from build123d import *

# Parameters (mm, degrees)
BOSS_EXTRUDE2_DEPTH = 15
SKETCH3_R           = 27
BOSS_EXTRUDE3_DEPTH = 46
SKETCH4_R           = 36
BOSS_EXTRUDE4_DEPTH = 38
MIRROR3_START       = 175
MIRROR3_OUTLINE_R   = 36
MIRROR3_DEPTH       = 53
MIRROR3_START_2     = 114
MIRROR3_2_DEPTH     = 15
MIRROR3_3_OUTLINE_R = 36
MIRROR3_3_DEPTH     = 15
MIRROR3_START_3     = 129
MIRROR3_4_OUTLINE_R = 27
MIRROR3_4_DEPTH     = 46


# Read off the part's stored shape, not the designer's step: Mirror3
with BuildPart() as part:
    # Sketch2 → Boss-Extrude2 (new body)
    with BuildSketch(Plane.XY):
        with BuildLine():
            Line((64.569893475, 47.23059238), (34.517510455, -54.224552409))
            ThreePointArc((34.517510455, -54.224552409), (0, -80), (-34.517510455, -54.224552409))
            Line((-34.517510455, -54.224552409), (-64.569893475, 47.23059238))
            ThreePointArc((-64.569893475, 47.23059238), (0, 80), (64.569893475, 47.23059238))
        make_face()
    boss_extrude2 = extrude(amount=BOSS_EXTRUDE2_DEPTH)

    # Sketch3 → Boss-Extrude3 (add)
    with BuildSketch(Plane.XY.offset(15)):
        with Locations((0, -44)):
            Circle(SKETCH3_R)
    extrude(amount=BOSS_EXTRUDE3_DEPTH)

    # Sketch4 → Boss-Extrude4 (add)
    with BuildSketch(Plane(origin=(0, 0, 0), x_dir=(-1, 0, 0), z_dir=(0, 0, -1))):
        Circle(SKETCH4_R)
    boss_extrude4 = extrude(amount=BOSS_EXTRUDE4_DEPTH)

    # Mirror2: Boss-Extrude2, Boss-Extrude4 across plane
    add(boss_extrude2.mirror(Plane.XY.offset(38)))
    add(boss_extrude4.mirror(Plane.XY.offset(38)))

    # Mirror3 2 outline → Mirror3 2 (add)
    with BuildSketch(Plane.XY.offset(MIRROR3_START_2)):
        with BuildLine():
            Line((-64.569893475, 47.23059238), (-34.517510455, -54.224552409))
            ThreePointArc((-34.517510455, -54.224552409), (0, -80), (34.517510455, -54.224552409))
            Line((34.517510455, -54.224552409), (64.569893475, 47.23059238))
            ThreePointArc((64.569893475, 47.23059238), (0, 80), (-64.569893475, 47.23059238))
        make_face()
    extrude(amount=MIRROR3_2_DEPTH)



with BuildPart() as body_2:
    # Mirror3 outline → Mirror3 (new body)
    with BuildSketch(Plane.XY.offset(MIRROR3_START)):
        Circle(MIRROR3_OUTLINE_R)
    extrude(amount=MIRROR3_DEPTH)

    # Mirror3 3 outline → Mirror3 3 (add)
    with BuildSketch(Plane.XY.offset(MIRROR3_START)):
        with BuildLine():
            Line((-64.569893475, 47.23059238), (-34.517510455, -54.224552409))
            ThreePointArc((-34.517510455, -54.224552409), (0, -80), (34.517510455, -54.224552409))
            Line((34.517510455, -54.224552409), (64.569893475, 47.23059238))
            ThreePointArc((64.569893475, 47.23059238), (0, 80), (-64.569893475, 47.23059238))
        make_face()
        Circle(MIRROR3_3_OUTLINE_R, mode=Mode.SUBTRACT)
    extrude(amount=MIRROR3_3_DEPTH)


with BuildPart() as part_1:
    add(part.part)

    add(body_2.part)  # Mirror3 4 merges body 2
    # Mirror3 4 outline → Mirror3 4 (add)
    with BuildSketch(Plane.XY.offset(MIRROR3_START_3)):
        with Locations((0, -44)):
            Circle(MIRROR3_4_OUTLINE_R)
    extrude(amount=MIRROR3_4_DEPTH)


solid = part_1.part
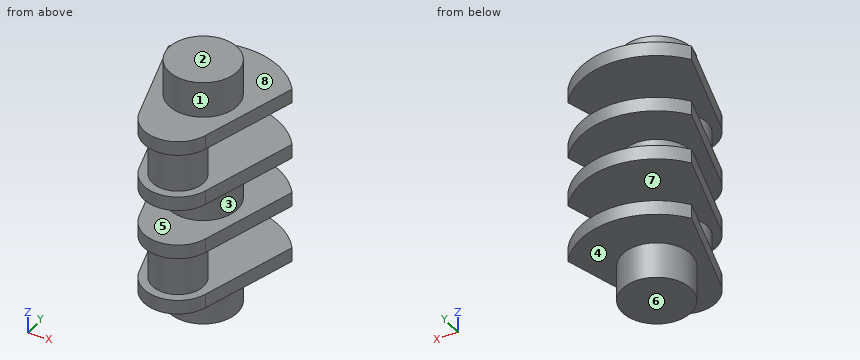
Could you check a few things on this model? Use its own coordinates, in mm. Face numbers are marked on the shaded views. A direction names the side the tool comes from. Round coordinates to 2 decimals unless told otherwise and drop trailing zeros. Order: outer loops, then holes, each group sorted by start corner. A loop starts at its lowest first (then second) coordinate and runs counter-clockwise, first axis right, second up.
Q1. Thinking about a two-plate mould opening in Z: for the marked faces 5, 6, 7 and 8, which applies, released by +Z, released by -Z, zero draft, split by the parting line, or undercut?
Geometry says:
face 5: undercut
face 6: released by -Z
face 7: undercut
face 8: released by +Z
Q2. Imagine slicing it at D-D, the plane y = -66.5. List the corners of the cut face in (x, z) for me, then the cut area to 3 significant figures.
Geometry says:
outline: (-28.1, 0) - (28.1, 0) - (28.1, 15) - (14.92, 15) - (14.92, 61) - (28.1, 61) - (28.1, 76) - (-28.1, 76) - (-28.1, 61) - (-14.92, 61) - (-14.92, 15) - (-28.1, 15) - close; (-28.1, 114) - (28.1, 114) - (28.1, 129) - (14.92, 129) - (14.92, 175) - (28.1, 175) - (28.1, 190) - (-28.1, 190) - (-28.1, 175) - (-14.92, 175) - (-14.92, 129) - (-28.1, 129) - close
area: 6,120 mm2
Q3. Imagine slicing it at B-B, the plane y = 68.5. List the corners of the cut face in (x, z) for me, then the cut area to 3 significant figures.
Geometry says:
outline: (-41.32, 0) - (41.32, 0) - (41.32, 15) - (-41.32, 15) - close; (-41.32, 61) - (41.32, 61) - (41.32, 76) - (-41.32, 76) - close; (-41.32, 114) - (41.32, 114) - (41.32, 129) - (-41.32, 129) - close; (-41.32, 175) - (41.32, 175) - (41.32, 190) - (-41.32, 190) - close
area: 4,960 mm2
Q4. Which directions (+Z, -Z, +X, -X, +Y, -Y) give clear straight access to the entire face, cutting with the end or side of a thin tool? Please do the marked faces 1, 2, 3 and 4.
Geometry says:
face 1: +Z
face 2: +Z, +X, -X, +Y, -Y
face 3: none
face 4: -Z
Q5. I'm going to push flat-ended pins straight in: P1, Ø4, axis at x = 42.5, z = 58, coming from the -Y side; P2, Ø3, axis at x = -0.5, z = 157, coming from the -Y side; P3, Ø12, axis at y = -39, z = 158.5, coming from the -X side; P4, Ø8, axis at x = -39, y = -33, coming from the -Z side. Where does each tip first touch, or does it pass through?
Geometry says:
P1: passes through
P2: stops at y = -71
P3: stops at x = -27
P4: stops at z = 0
Q6. Imagine slicing it at C-C, the plane z = 135. List the corners of the cut face in (x, y) for me, then the cut area to 3 significant figures.
Geometry says:
outline: circle Ø54 at (0, -44)
area: 2,290 mm2
Q7. Please list where these lines run through material, in increasing order: probe 1 along Z at (x, y) = (9.5, 4); probe 2 along Z at (x, y) = (-36, 44); probe 3 along Z at (x, y) = (18, -51).
Geometry says:
probe 1: z = -38 to 15, 61 to 129, 175 to 228
probe 2: z = 0 to 15, 61 to 76, 114 to 129, 175 to 190
probe 3: z = 0 to 76, 114 to 190
Q8. Imagine slicing it at A-A, the plane y = -13. List the corners of the cut face in (x, z) for me, then the cut area to 3 significant figures.
Geometry says:
outline: (-46.73, 0) - (-33.57, 0) - (-33.57, -38) - (33.57, -38) - (33.57, 0) - (46.73, 0) - (46.73, 15) - (-46.73, 15) - close; (-46.73, 61) - (46.73, 61) - (46.73, 76) - (33.57, 76) - (33.57, 114) - (46.73, 114) - (46.73, 129) - (-46.73, 129) - (-46.73, 114) - (-33.57, 114) - (-33.57, 76) - (-46.73, 76) - close; (-46.73, 175) - (46.73, 175) - (46.73, 190) - (33.57, 190) - (33.57, 228) - (-33.57, 228) - (-33.57, 190) - (-46.73, 190) - close
area: 13,300 mm2
